Source: CAD feature listing. Evaluate the final solid. Frame: model axes, mm. Give positions to 0.01 mm unless a question says otherwise; leave off trailing zeros. Order: outer loops, then holes, each group sorted by start corner. A loop starts at its lowest first (then second) coordinate and runs counter-clockwise, first axis right, second up. Notation, with made-up numbers: (-27.75, 37.25) - (14.25, 37.25) arc R23 ccw to (14.25, 54.25) - close; hole circle Ø8 at (-15, 35). An arc over 180 degrees is marked (long way). Write each question's results on one line, items separated by ' | '. Start each with the question number.
Item 1: Section C-C on z = 31.5. Output: boundary loops of the cut face in (x, y), and give its area (3 significant figures).
Item 2: Line query: line 1 along Z through (x, y) = (-6.7, 0.75); line 2 along X through (y, z) = (-2.25, 14); line 3 along Z through (x, y) = (-5.25, -2). Output: solid intervals per line, ascending.
Item 3: Contact query for flat-ended pins moving along their axis: pin 1 Ø3 at (x, z) = (-1, 60) entering from +Y; pin 2 Ø1.6 at (y, z) = (2, 56) entering from -X; pin 3 Ø6.5 at (x, z) = (-6.7, 14) entering from -Y; pin 4 Ø1.6 at (y, z) = (1.5, 91.5) entering from +X. Output: stop coordinate, or through.
Item 4: Section A-A on z = 14. Output: boundary loops of the cut face in (x, y), and give its area (3 significant figures).
Item 5: Section B-B on y = -3. Output: boundary loops of the cut face in (x, z), and give its area (3 significant figures).
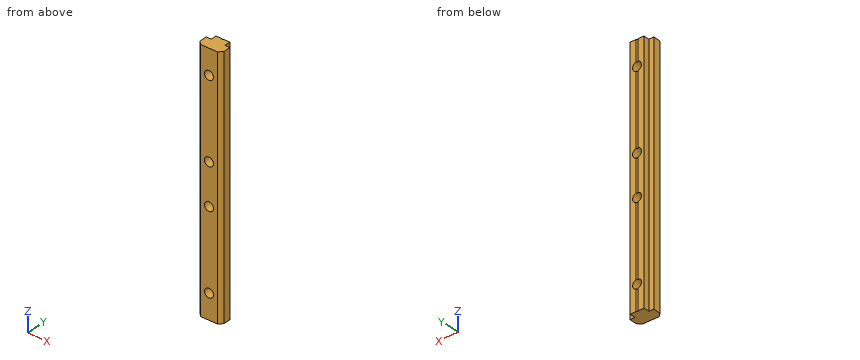
```python
from build123d import *

# Parameters (mm, degrees)
EXTRUDE_1_DEPTH        = 140
HOLE_WIZARD_M6_1_D     = 5
HOLE_WIZARD_M6_1_DEPTH = 28
HOLE_WIZARD_M6_1_TIP   = 1.502151548


with BuildPart() as part:
    # 草图1 → 凸台-拉伸1 (new body)
    with BuildSketch(Plane.XY):
        Polygon((-2, -6.2), (-11.4, -6.2), (-13.4, -4.2), (-13.4, 0), (-10.6, 0), (-10.6, 3.3), (-7.2, 3.3), (-6.7, 2.8), (-6.2, 3.3), (-2.8, 3.3), (-2.8, 0), (0, 0), (0, -4.2), align=None)
    extrude(amount=EXTRUDE_1_DEPTH)

    # M6 螺纹孔1
    with Locations(Plane(origin=(-6.7, -6.2, 14), x_dir=(-1, 0, 0), z_dir=(0, -1, 0))):
        with Locations((0, 0), (0, -44.5), (0, -67.5), (0, -112)):
            Hole(HOLE_WIZARD_M6_1_D / 2, depth=HOLE_WIZARD_M6_1_DEPTH)
            with Locations((0, 0, -(HOLE_WIZARD_M6_1_DEPTH + HOLE_WIZARD_M6_1_TIP / 2))):  # 118° drill point
                Cone(0, HOLE_WIZARD_M6_1_D / 2, HOLE_WIZARD_M6_1_TIP, mode=Mode.SUBTRACT)


solid = part.part
```
Evaluation:
1) outline: (-13.4, -4.2) - (-11.4, -6.2) - (-2, -6.2) - (0, -4.2) - (0, 0) - (-2.8, 0) - (-2.8, 3.3) - (-6.2, 3.3) - (-6.7, 2.8) - (-7.2, 3.3) - (-10.6, 3.3) - (-10.6, 0) - (-13.4, 0) - close | area: 105 mm^2
2) line 1: z = 0 to 11.5, 16.5 to 56, 61 to 79, 84 to 123.5, 128.5 to 140 | line 2: x = -13.4 to -9.2, -4.2 to 0 | line 3: z = 0 to 11.96, 16.04 to 56.46, 60.54 to 79.46, 83.54 to 123.96, 128.04 to 140
3) pin 1: stops at y = 0 | pin 2: stops at x = -10.6 | pin 3: stops at y = -6.2 | pin 4: stops at x = -2.8
4) outline: (-13.4, -4.2) - (-11.4, -6.2) - (-9.2, -6.2) - (-9.2, 3.3) - (-10.6, 3.3) - (-10.6, 0) - (-13.4, 0) - close; (-4.2, -6.2) - (-2, -6.2) - (0, -4.2) - (0, 0) - (-2.8, 0) - (-2.8, 3.3) - (-4.2, 3.3) - close | area: 57.3 mm^2
5) outline: (-13.4, 0) - (0, 0) - (0, 140) - (-13.4, 140) - close; hole circle Ø5 at (-6.7, 14); hole circle Ø5 at (-6.7, 58.5); hole circle Ø5 at (-6.7, 81.5); hole circle Ø5 at (-6.7, 126) | area: 1,800 mm^2
